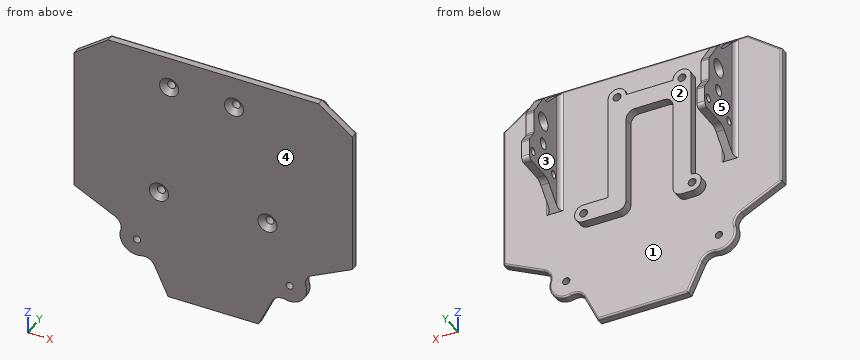
from build123d import *

# Parameters (mm, degrees)
BOSS_EXTRUDE1_DEPTH = 3.5
SKETCH2_W           = 3.5
SKETCH2_H           = 36.5
BOSS_EXTRUDE2_DEPTH = 25
CHAMFER1_SIZE       = 10
FILLET1_R           = 2
SKETCH3_R           = 1.75
CUT_EXTRUDE1_DEPTH  = 108
FILLET2_R           = 2
SKETCH4_R           = 4
SKETCH4_R_2         = 2.5
CUT_EXTRUDE2_DEPTH  = 108
CUT_EXTRUDE3_DEPTH  = 108
FILLET3_R           = 2
FILLET4_R           = 5
SKETCH6_R           = 1.75
BOSS_EXTRUDE3_DEPTH = 4
SKETCH7_R           = 1.75
CUT_EXTRUDE4_DEPTH  = 37
CHAMFER2_SIZE       = 2.5
CHAMFER2_SIZE2      = 2
CUT_EXTRUDE5_DEPTH  = 37
SKETCH9_R           = 1.6
BOSS_EXTRUDE4_DEPTH = 3.5
FILLET5_R           = 5
FILLET6_R           = 0.75


with BuildPart() as part:
    # Sketch1 → Boss-Extrude1 (new body)
    with BuildSketch(Plane(origin=(0, 0, 0), x_dir=(1, 0, 0), z_dir=(0, 1, 0))):
        Polygon((0, 0), (63, 0), (93, 0), (93, 75), (63, 90), (51.5, 115), (31.5, 115), (11.5, 115), (0, 90), (-30, 75), (-30, 0), align=None)
    extrude(amount=BOSS_EXTRUDE1_DEPTH)

    # Sketch2 → Boss-Extrude2 (add)
    with BuildSketch(Plane(origin=(0, 3.5, 0), x_dir=(1, 0, 0), z_dir=(0, 1, 0))):
        with Locations((-7.267018522, 29.254092769)):
            Rectangle(SKETCH2_W, SKETCH2_H)
        with Locations((70.267018522, 29.254092769)):
            Rectangle(SKETCH2_W, SKETCH2_H)
    extrude(amount=BOSS_EXTRUDE2_DEPTH)

    # Chamfer1
    chamfer1_edges = [part.edges().sort_by_distance(p)[0] for p in [
        (-7.267018522, 3.5, -11.004092769),
        (-7.267018522, 3.5, -47.504092769),
        (70.267018522, 3.5, -11.004092769),
        (70.267018522, 3.5, -47.504092769),
    ]]
    chamfer(chamfer1_edges, length=CHAMFER1_SIZE)

    # Fillet1
    fillet1_edges = [part.edges().sort_by_distance(p)[0] for p in [
        (-5.517018522, 3.5, -29.254092769),
        (68.517018522, 3.5, -29.254092769),
    ]]
    fillet(fillet1_edges, radius=FILLET1_R)

    # Sketch3 → Cut-Extrude1 (cut)
    with BuildSketch(Plane(origin=(72.017018522, 0, 0), x_dir=(0, 0, -1), z_dir=(1, 0, 0))):
        with Locations((42.33980963, 25.5)):
            Circle(SKETCH3_R)
        with Locations((42.33980963, 8)):
            Circle(SKETCH3_R)
    extrude(amount=-CUT_EXTRUDE1_DEPTH, mode=Mode.SUBTRACT)

    # Fillet2
    fillet2_edges = [part.edges().sort_by_distance(p)[0] for p in [
        (-9.017018522, 3.5, -29.254092769),
        (72.017018522, 3.5, -29.254092769),
    ]]
    fillet(fillet2_edges, radius=FILLET2_R)

    # Sketch4 → Cut-Extrude2 (cut)
    with BuildSketch(Plane(origin=(72.017018522, 0, 0), x_dir=(0, 0, -1), z_dir=(1, 0, 0))):
        with Locations((22.33980963, 16.75)):
            Circle(SKETCH4_R)
        with Locations((33.03980963, 16.75)):
            Circle(SKETCH4_R_2)
    extrude(amount=-CUT_EXTRUDE2_DEPTH, mode=Mode.SUBTRACT)

    # Sketch5 → Cut-Extrude3 (cut)
    with BuildSketch(Plane(origin=(72.017018522, 0, 0), x_dir=(0, 0, -1), z_dir=(1, 0, 0))):
        Polygon((22.33980963, 24.747503661), (11.004092769, 16.75), (11.004092769, 28.5), (38.0603401, 28.5), (33.03980963, 24.747503661), align=None)
    extrude(amount=-CUT_EXTRUDE3_DEPTH, mode=Mode.SUBTRACT)

    # Fillet3
    fillet3_edges = [part.edges().sort_by_distance(p)[0] for p in [
        (70.267018522, 28.5, -38.0603401),
        (-7.267018522, 24.747503661, -33.03980963),
        (70.267018522, 24.747503661, -33.03980963),
        (-7.267018522, 24.747503661, -22.33980963),
        (70.267018522, 24.747503661, -22.33980963),
        (-7.267018522, 28.5, -38.0603401),
        (-7.267018522, 16.75, -11.004092769),
        (70.267018522, 16.75, -11.004092769),
        (-7.267018522, 28.5, -47.504092769),
        (70.267018522, 28.5, -47.504092769),
        (-7.267018522, 13.5, -11.004092769),
        (70.267018522, 13.5, -11.004092769),
    ]]
    fillet(fillet3_edges, radius=FILLET3_R)

    # Fillet4
    fillet4_edges = [part.edges().sort_by_distance(p)[0] for p in [
        (-7.267018522, 13.5, -47.504092769),
        (70.267018522, 13.5, -47.504092769),
    ]]
    fillet(fillet4_edges, radius=FILLET4_R)

    # Sketch6 → Boss-Extrude3 (add)
    with BuildSketch(Plane(origin=(0, 3.5, 0), x_dir=(1, 0, 0), z_dir=(0, 1, 0))):
        with BuildLine():
            ThreePointArc((8, 14), (12, 10), (16, 14))
            Line((16, 14), (36.7, 14))
            ThreePointArc((36.7, 14), (40.7, 10), (44.7, 14))
            Line((44.7, 14), (44.7, 61))
            Line((44.7, 61), (55.5, 61))
            ThreePointArc((55.5, 61), (59.5, 65), (55.5, 69))
            Line((55.5, 69), (40.7, 69))
            ThreePointArc((40.7, 69), (37.871572875, 67.828427125), (36.7, 65))
            Line((36.7, 65), (36.7, 26))
            ThreePointArc((36.7, 26), (35.528427125, 23.171572875), (32.7, 22))
            Line((32.7, 22), (20, 22))
            ThreePointArc((20, 22), (17.171572875, 23.171572875), (16, 26))
            Line((16, 26), (16, 66))
            ThreePointArc((16, 66), (14.828427125, 68.828427125), (12, 70))
            Line((12, 70), (7.5, 70))
            ThreePointArc((7.5, 70), (3.5, 66), (7.5, 62))
            ThreePointArc((7.5, 62), (7.856858863, 61.606355585), (8, 61.09467718))
            ThreePointArc((8, 61.09467718), (8.000969427, 61.04733859), (8, 61))
            Line((8, 61), (8, 14))
        make_face()
        with Locations((12, 14)):
            Circle(SKETCH6_R, mode=Mode.SUBTRACT)
        with Locations((40.7, 14)):
            Circle(SKETCH6_R, mode=Mode.SUBTRACT)
        with Locations((7.5, 66)):
            Circle(SKETCH6_R, mode=Mode.SUBTRACT)
        with Locations((55.5, 65)):
            Circle(SKETCH6_R, mode=Mode.SUBTRACT)
    extrude(amount=BOSS_EXTRUDE3_DEPTH)

    # Sketch7 → Cut-Extrude4 (cut)
    with BuildSketch(Plane(origin=(0, 7.5, 0), x_dir=(1, 0, 0), z_dir=(0, 1, 0))):
        with Locations((7.5, 66)):
            Circle(SKETCH7_R)
        with Locations((55.5, 65)):
            Circle(SKETCH7_R)
        with Locations((40.7, 14)):
            Circle(SKETCH7_R)
        with Locations((12, 14)):
            Circle(SKETCH7_R)
    extrude(amount=-CUT_EXTRUDE4_DEPTH, mode=Mode.SUBTRACT)

    # Chamfer2
    chamfer2_edges = [part.edges().sort_by_distance(p)[0] for p in [
        (5.75, 0, -66),
        (53.75, 0, -65),
        (38.95, 0, -14),
        (10.25, 0, -14),
    ]]
    chamfer2_side = [part.faces().sort_by_distance(p)[0] for p in [
        (31.50834927, 0, -49.636894868),
    ]]
    chamfer(chamfer2_edges, length=CHAMFER2_SIZE, length2=CHAMFER2_SIZE2, reference=chamfer2_side[0])

    # Sketch8 → Cut-Extrude5 (cut)
    with BuildSketch(Plane(origin=(0, 3.5, 0), x_dir=(1, 0, 0), z_dir=(0, 1, 0))):
        Polygon((-30, 11.112303486), (-15, 0), (-30, 0), align=None)
        Polygon((78, 0), (93, 11.004092769), (93, 0), align=None)
    extrude(amount=-CUT_EXTRUDE5_DEPTH, mode=Mode.SUBTRACT)

    # Sketch9 → Boss-Extrude4 (add)
    with BuildSketch(Plane(origin=(0, 3.5, 0), x_dir=(1, 0, 0), z_dir=(0, 1, 0))):
        with BuildLine():
            Line((-7.230389166, 86.384805417), (0, 90))
            Line((0, 90), (3.257553694, 97.081638464))
            ThreePointArc((3.257553694, 97.081638464), (-7.613842407, 97.250752983), (-7.230389166, 86.384805417))
        make_face()
        with Locations((-2.258509261, 92)):
            Circle(SKETCH9_R, mode=Mode.SUBTRACT)
        with BuildLine():
            Line((59.742446306, 97.081638464), (63, 90))
            Line((63, 90), (70.230389166, 86.384805417))
            ThreePointArc((70.230389166, 86.384805417), (70.613842407, 97.250752983), (59.742446306, 97.081638464))
        make_face()
        with Locations((65.258509261, 92)):
            Circle(SKETCH9_R, mode=Mode.SUBTRACT)
    extrude(amount=-BOSS_EXTRUDE4_DEPTH)

    # Fillet5
    fillet5_edges = [part.edges().sort_by_distance(p)[0] for p in [
        (3.257553694, 1.75, -97.081638464),
        (-7.230389166, 1.75, -86.384805417),
        (70.230389166, 1.75, -86.384805417),
        (59.742446306, 1.75, -97.081638464),
    ]]
    fillet(fillet5_edges, radius=FILLET5_R)

    # Fillet6
    fillet6_edges = [part.edges().sort_by_distance(p)[0] for p in [
        (84.006223284, 3.5, -79.496888358),
        (31.5, 3.5, -115),
        (8.506790147, 3.5, -108.493022059),
        (-30, 3.5, -43.056151743),
        (31.5, 3.5, 0),
        (-22.5, 3.5, -5.556151743),
        (93, 3.5, -43.002046385),
        (85.5, 3.5, -5.502046385),
        (70.628471691, 3.5, -97.235790627),
        (54.493209853, 3.5, -108.493022059),
        (-7.628471691, 3.5, -97.235790627),
        (-21.006223284, 3.5, -79.496888358),
        (59.902970742, 3.5, -99.550028659),
        (72.663421616, 3.5, -86.47169031),
        (3.097029258, 3.5, -99.550028659),
        (-9.663421616, 3.5, -86.47169031),
    ]]
    fillet(fillet6_edges, radius=FILLET6_R)


solid = part.part
For this review, take the finished solid that the model builds, in its own axes (mm). Face numbers are marked on the shaded views. A direction names the side the tool comes from. Give positions to 0.01 mm unless a question says otherwise; leave off trailing zeros. Loops run counter-clockwise (first coordinate to the right, second up) from the corner with the lowest first, then second, coordinate; pieces in that order, holes last.
Item 1: Take a section at A-A, the plane x = 23. State the section outline as (y, z) points, and give its area (3 significant figures).
Item 2: For line 1 along X through (y, z) = (1.8, -92); line 2 along Z through (x, y) = (12, 4.25); line 3 along X through (y, z) = (6.1, -66), list the stretches that pass through material, from the lowest coordinate up.
Item 3: Draft analysis for pull direction X (two halves, no side actions). For the marked faces 3, 4 and 5, state which applies: +X half, -X half, draft (parallel to the pull), parting line (faces both ways), or undercut.
Item 4: Insertion check: pin 1 (13 mm diameter, centred on y = 16.75, z = -22.34, fed in from +X); pin 2 (4 mm diameter, centred on x = 55.5, z = -65, fed in from +Y); pin 3 (3 mm diameter, centred on x = 12, z = -14, fed in from -Y); pin 4 (7 mm diameter, centred on y = 12.5, z = -20, fed in from -X). Each pin has a flat end and moves straight along its axis. Give the tip position at first contact, or say it passes through.
Item 5: Take a section at B-B, the plane z = -92. Give the number of separate pieces and of enclosed holes in the cut face, and give its area (3 significant figures).
Item 6: Tool access review of the marked faces 1 and 2: name each direction out of +Z, -Z, +X, -X, +Y, -Y from which nothing blocks a thin tool from reaching the whole face with its end or side.
Calculated:
1. outline: (0, -115) - (2.75, -115) arc R0.75 ccw to (3.5, -114.25) - (3.5, -22) - (7.5, -22) - (7.5, -14) - (3.5, -14) - (3.5, -0.75) arc R0.75 ccw to (2.75, 0) - (0, 0) - close
1. area: 434 mm2
2. line 1: x = -9.76 to -3.86, -0.66 to 63.66, 66.86 to 72.76
2. line 2: z = -70 to -15.75, -12.25 to -10
2. line 3: x = 3.5 to 5.75, 9.25 to 16, 36.83 to 54.06, 56.94 to 59.37
3. face 3: undercut
3. face 4: draft
3. face 5: -X half
4. pin 1: stops at x = 72.02
4. pin 2: stops at y = 7.5
4. pin 3: passes through
4. pin 4: stops at x = -9.02
5. separate pieces: 3
5. enclosed holes: 0
5. area: 266 mm2
6. face 1: +Y
6. face 2: +Z, -Z, +Y
